Model file for the job. Use its own axes, mm. A direction names the side the tool comes from. Give positions to 0.01 mm unless a question says otherwise; leave off trailing zeros. Loops run counter-clockwise (first coordinate to the right, second up) from the corner with the lowest first, then second, coordinate; pieces in that order, holes last. Notation, with made-up numbers: (3, 23.5) - (57, 23.5) arc R14 ccw to (57, 33.5) - close; hole circle Ø1 at (-4, 28.25). An arc over 180 degrees is marked (long way). Use a Markdown table: item, result.
from build123d import *

# Parameters (mm, degrees)
BOSS_EXTRUDE1_DEPTH = 36
SKETCH2_R           = 1.6
CUT_EXTRUDE1_DEPTH  = 5
FILLET1_R           = 5


with BuildPart() as part:
    # Sketch1 → Boss-Extrude1 (new body)
    with BuildSketch(Plane.XY):
        with BuildLine():
            Line((-19.2, 0), (-19.2, -16.8))
            Line((-19.2, -16.8), (-49.2, -16.8))
            Line((-49.2, -16.8), (-49.2, -11.8))
            Line((-49.2, -11.8), (-24.2, -11.8))
            Line((-24.2, -11.8), (-24.2, 0))
            ThreePointArc((-24.2, 0), (0, 24.2), (24.2, 0))
            Line((24.2, 0), (24.2, -11.8))
            Line((24.2, -11.8), (49.2, -11.8))
            Line((49.2, -11.8), (49.2, -16.8))
            Line((49.2, -16.8), (19.2, -16.8))
            Line((19.2, -16.8), (19.2, 0))
            ThreePointArc((19.2, 0), (0, 19.2), (-19.2, 0))
        make_face()
    extrude(amount=-BOSS_EXTRUDE1_DEPTH)

    # Sketch2 → Cut-Extrude1 (cut)
    with BuildSketch(Plane(origin=(0, -11.8, 0), x_dir=(1, 0, 0), z_dir=(0, 1, 0))):
        with Locations((-36.7, 27)):
            Circle(SKETCH2_R)
        with Locations((-36.7, 9)):
            Circle(SKETCH2_R)
        with Locations((36.7, 27)):
            Circle(SKETCH2_R)
        with Locations((36.7, 9)):
            Circle(SKETCH2_R)
    extrude(amount=-CUT_EXTRUDE1_DEPTH, mode=Mode.SUBTRACT)

    # Fillet1
    fillet1_edges = [part.edges().sort_by_distance(p)[0] for p in [
        (24.2, -11.8, -18),
        (-24.2, -11.8, -18),
    ]]
    fillet(fillet1_edges, radius=FILLET1_R)


solid = part.part
(1) Slice it at A-A, the plane z = -27. Write the cut outline in (x, y).
Computed:
| item | result |
|---|---|
| outline | (-49.2, -16.8) - (-38.3, -16.8) - (-38.3, -11.8) - (-49.2, -11.8) - close; (-35.1, -16.8) - (-19.2, -16.8) - (-19.2, 0) arc R19.2 cw to (19.2, 0) - (19.2, -16.8) - (35.1, -16.8) - (35.1, -11.8) - (29.2, -11.8) arc R5 cw to (24.2, -6.8) - (24.2, 0) arc R24.2 ccw to (-24.2, 0) - (-24.2, -6.8) arc R5 cw to (-29.2, -11.8) - (-35.1, -11.8) - close; (38.3, -16.8) - (49.2, -16.8) - (49.2, -11.8) - (38.3, -11.8) - close |
(2) 3-axis set-ups, long thin cutter, end or side, ignore diameter. For faces 4 (the flat face through (-24.2, -3, -18)), 5 (the flat face through (24.2, -3, -18)), 6 (the flat face through (-34, -16.8, -18)), 7 (the flat face through (19.2, -9, -18)), 8 (the cylindrical face through (-35.22, -14.26, -8.39)): which of +Z, -Z, +X, -X, +Y, -Y reach the whole face in a straight line?
Computed:
| item | result |
|---|---|
| face 4 | +Z, -Z, -X, +Y |
| face 5 | +Z, -Z, +X, +Y |
| face 6 | +Z, -Z, +X, -X, -Y |
| face 7 | +Z, -Z, -Y |
| face 8 | +Y, -Y |
(3) Slice it at C-C, the plane x = 36.7. Write the cut outline in (y, z).
Computed:
| item | result |
|---|---|
| outline | (-16.8, -36) - (-11.8, -36) - (-11.8, -28.6) - (-16.8, -28.6) - close; (-16.8, -25.4) - (-11.8, -25.4) - (-11.8, -10.6) - (-16.8, -10.6) - close; (-16.8, -7.4) - (-11.8, -7.4) - (-11.8, 0) - (-16.8, 0) - close |
(4) Slice it at D-D, the plane z = -20.5. Write the cut outline in (x, y).
Computed:
| item | result |
|---|---|
| outline | (-49.2, -16.8) - (-19.2, -16.8) - (-19.2, 0) arc R19.2 cw to (19.2, 0) - (19.2, -16.8) - (49.2, -16.8) - (49.2, -11.8) - (29.2, -11.8) arc R5 cw to (24.2, -6.8) - (24.2, 0) arc R24.2 ccw to (-24.2, 0) - (-24.2, -6.8) arc R5 cw to (-29.2, -11.8) - (-49.2, -11.8) - close |
(5) Slice it at B-B, the plane y = -1. Write the cut outline in (x, z), plus the area to 3 significant figures.
Computed:
| item | result |
|---|---|
| outline | (-24.2, -36) - (-19.2, -36) - (-19.2, 0) - (-24.2, 0) - close; (19.2, -36) - (24.2, -36) - (24.2, 0) - (19.2, 0) - close |
| area | 360 mm² |
(6) Pin check, flat tips, straight feed: P1, Ø8, axis at x = 13, z = -17, coming from the +Y side; P2, Ø7.5, axis at y = -2, z = -13.5, coming from the -X side; P3, Ø18.5, axis at y = -8.5, z = -22, coming from the +X side; P4, Ø5, axis at x = -36.7, z = -27, coming from the +Y side. Stop position of each tip, or through.
Computed:
| item | result |
|---|---|
| P1 | y = 22.46 |
| P2 | x = -24.2 |
| P3 | x = 49.2 |
| P4 | y = -11.8 |
(7) Drill centre lines: probe 1 along X at (y, z) = (-14.3, -27); probe 2 along Z at (x, y) = (36.7, -14.4); probe 3 along X at (y, z) = (-4.5, -29). Where is each one in solid material? Low to high. Write a range as [from, to].
Computed:
| item | result |
|---|---|
| probe 1 | [-49.2, -38.3], [-35.1, -19.2], [19.2, 35.1], [38.3, 49.2] |
| probe 2 | [-36, -28.6], [-25.4, -10.6], [-7.4, 0] |
| probe 3 | [-24.2, -19.2], [19.2, 24.2] |
(8) Mould opens along Z. For faces 1 (the cylindrical face through (25.63, -10.3, -18.25)), 2 (the cylindrical face through (35.1, -14.26, -27.07)), 3 (the flat face through (11, 16, -36)) say: pulls with the +Z half, pulls with the -Z half, needs draft (parallel to the pull), parting line crosses it, or undercut.
Computed:
| item | result |
|---|---|
| face 1 | needs draft |
| face 2 | undercut |
| face 3 | pulls with the -Z half |
